Here's how the part is built. I have some questions about the finished solid (model axes, mm). A direction names the side the tool comes from. Coordinates: 2 decimals unless noted, no trailing zeros. Loops run counter-clockwise (first coordinate to the right, second up) from the corner with the lowest first, then second, coordinate; pieces in that order, holes last. Notation, with made-up numbers: (58, 7.25) -> (74, 7.25) arc R37 ccw to (74, 44.25) -> close; hole circle Ø10 at (7.25, 6). An arc over 180 degrees is marked (long way). Answer as a JSON object with one key per item and string values. Group by question number.
Q1. I want a section at A-A on x = 0. Write out the boundary of the cut face in (y, z) (3 decimals).
Q2. On a 3-axis mill with a long thin cutter (end or side, diameter ignored), from which of +Z, -Z, +X, -X, +Y, -Y can I reach the whole of each face in a straight line? I mean faces 4 (the flat face through (25.4, 70, 7)), 5 (the flat face through (0, 93, 7.5)), 6 (the flat face through (-1, -1, 13.625)). Say none if no direction works.
Q3. I need wall thicknesses on line 1 (Y direction, x = 11.25, z = 6.25); line 2 (Y direction, x = -1.5, z = 19.75); line 3 (Z direction, x = 12.5, y = -35) (3 decimals). Which ranges of each line are inside material? Lowest first, please.
Q4. I want a section at D-D on z = 5.75. Write out the boundary of the cut face in (x, y).
Q5. Thinking about a two-plate mould opening in Y: for faces 1 (the cylindrical face through (-1.71, -47.47, 18.56)), 2 (the cylindrical face through (-34.783, 18.75, 18.555)), 3 (the flat face through (-25.4, 70, 7)), which applies, released by +Y, released by -Y, zero draft, split by the parting line, or undercut?
Q6. I want a section at B-B on y = 18.64. Write out the boundary of the cut face in (x, z) (3 decimals).
Q7. I want a section at C-C on y = 37.28. Write out the boundary of the cut face in (x, z) (3 decimals), then the cut area to 3 significant figures.
Q8. I'm going to push flat-ended pins straight in: pin 1 (8 mm diameter, centred on x = 5.5, z = 10, fed in from -Y); pin 2 (11 mm diameter, centred on x = 1, z = 4, fed in from -Y); pin 3 (8 mm diameter, centred on x = -6.5, y = 8.5, fed in from -Z) (3 decimals); pin 4 (4.5 mm diameter, centred on x = -32.29, y = -18.64, fed in from -Z). Where does each tip first touch, or does it pass through?
```python
from build123d import *

# Parameters (mm, degrees)
SKETCH1_W           = 50.8
SKETCH1_H           = 65.000000038
SKETCH1_R           = 2.5
EXTRUDE_5_DEPTH     = 7.5
SKETCH1_3_W         = 50.8
SKETCH1_3_H         = 10
BOSS_EXTRUDE1_DEPTH = 13.625
BOSS_EXTRUDE2_START = 13.625
SKETCH1_4_R         = 2.5
SKETCH1_4_W         = 50.8
SKETCH1_4_H         = 10
BOSS_EXTRUDE2_DEPTH = 10
CHAMFER1_SIZE       = 10
CHAMFER1_SIZE_2     = 27.474774195
FILLET1_R           = 5


with BuildPart() as part:
    # Sketch1 → 5 (new body)
    with BuildSketch(Plane.XY):
        with Locations((0, 87.638385637)):
            Rectangle(SKETCH1_W, SKETCH1_H)
        with Locations((-11.25, 70.138385656)):
            Circle(SKETCH1_R, mode=Mode.SUBTRACT)
        with Locations((-11.25, 105.138385656)):
            Circle(SKETCH1_R, mode=Mode.SUBTRACT)
        with Locations((11.25, 70.138385656)):
            Circle(SKETCH1_R, mode=Mode.SUBTRACT)
        with Locations((11.25, 105.138385656)):
            Circle(SKETCH1_R, mode=Mode.SUBTRACT)
    extrude(amount=EXTRUDE_5_DEPTH)

    # Sketch1<3> → Boss-Extrude1 (add)
    with BuildSketch(Plane.XY):
        with Locations((0, 50.138385618)):
            Rectangle(SKETCH1_3_W, SKETCH1_3_H)
    extrude(amount=BOSS_EXTRUDE1_DEPTH)

    # Sketch1<4> → Boss-Extrude2 (add)
    # profile 1 of 2: a face of its own
    with BuildSketch(Plane.XY.offset(BOSS_EXTRUDE2_START)):
        with BuildLine():
            Line((-25.4, 45.138385618), (-25.4, 40.138385618))
            ThreePointArc((-25.4, 40.138385618), (0, -47.5), (25.4, 40.138385618))
            Line((25.4, 40.138385618), (25.4, 45.138385618))
            Line((25.4, 45.138385618), (-25.4, 45.138385618))
        make_face()
        with Locations((-32.285427053, -18.64)):
            Circle(SKETCH1_4_R, mode=Mode.SUBTRACT)
        with Locations((-32.285427053, 18.64)):
            Circle(SKETCH1_4_R, mode=Mode.SUBTRACT)
        with Locations((0, -37.28)):
            Circle(SKETCH1_4_R, mode=Mode.SUBTRACT)
        with Locations((32.285427053, -18.64)):
            Circle(SKETCH1_4_R, mode=Mode.SUBTRACT)
        with Locations((32.285427053, 18.64)):
            Circle(SKETCH1_4_R, mode=Mode.SUBTRACT)
        with Locations((0, 37.28)):
            Circle(SKETCH1_4_R, mode=Mode.SUBTRACT)
    # profile 2 of 2: a face of its own
    with BuildSketch(Plane.XY.offset(BOSS_EXTRUDE2_START)):
        with Locations((0, 50.138385618)):
            Rectangle(SKETCH1_4_W, SKETCH1_4_H)
    extrude(amount=BOSS_EXTRUDE2_DEPTH)

    # Chamfer1
    # the kernel refuses this chamfer: 27.474774195, 10 mm, written as the material it adds along each edge
    with BuildSketch(Plane(origin=(-25.4, 55.138385618, 7.5), x_dir=(0, 0.9950833631817486, -0.0990409022520505), z_dir=(1, 0, 0))) as chamfer1_piece_1_section:
        Polygon((CHAMFER1_SIZE * 0.995083363182, CHAMFER1_SIZE * 0.0990409022521), (-CHAMFER1_SIZE_2 * 0.0990409022504, CHAMFER1_SIZE_2 * 0.995083363165), (0, 0), align=None)
    chamfer1_piece_1 = extrude(amount=50.8, mode=Mode.PRIVATE)
    chamfer1_piece_1 = split(chamfer1_piece_1, bisect_by=Plane(origin=(0, 58.7545268, 23.625), z_dir=(0, 0, -1)), keep=Keep.TOP, mode=Mode.PRIVATE)
    add(chamfer1_piece_1)

    # Fillet1
    fillet1_edges = [part.edges().sort_by_distance(p)[0] for p in [
        (0, 59.26936559, 23.625),
    ]]
    fillet(fillet1_edges, radius=FILLET1_R)


solid = part.part
```
Result set:
{
 "1": {"outline": "(-47.5, 13.625) -> (-39.78, 13.625) -> (-39.78, 23.625) -> (-47.5, 23.625) -> close; (-34.78, 13.625) -> (34.78, 13.625) -> (34.78, 23.625) -> (-34.78, 23.625) -> close; (39.78, 13.625) -> (45.138, 13.625) -> (45.138, 0) -> (120.138, 0) -> (120.138, 7.5) -> (65.138, 7.5) -> (60.467, 20.335) arc R5 ccw to (55.768, 23.625) -> (39.78, 23.625) -> close"},
 "2": {"face 4": "+Z, -Z, +X, +Y", "face 5": "+Z, +X, -X, +Y", "face 6": "-Z, +X, -X, -Y"},
 "3": {"line 1": "y = 45.14 to 67.64, 72.64 to 102.64, 107.64 to 120.14", "line 2": "y = -47.48 to -39.28, -35.28 to 35.28, 39.28 to 60.68", "line 3": "z = 13.625 to 23.625"},
 "4": {"outline": "(-25.4, 45.14) -> (25.4, 45.14) -> (25.4, 120.14) -> (-25.4, 120.14) -> close; hole circle Ø5 at (-11.25, 70.14); hole circle Ø5 at (-11.25, 105.14); hole circle Ø5 at (11.25, 70.14); hole circle Ø5 at (11.25, 105.14)"},
 "5": {"face 1": "split by the parting line", "face 2": "undercut", "face 3": "zero draft"},
 "6": {"outline": "(-43.69, 13.625) -> (-34.785, 13.625) -> (-34.785, 23.625) -> (-43.69, 23.625) -> close; (-29.785, 13.625) -> (29.785, 13.625) -> (29.785, 23.625) -> (-29.785, 23.625) -> close; (34.785, 13.625) -> (43.69, 13.625) -> (43.69, 23.625) -> (34.785, 23.625) -> close"},
 "7": {"outline": "(-29.436, 13.625) -> (-2.5, 13.625) -> (-2.5, 23.625) -> (-29.436, 23.625) -> close; (2.5, 13.625) -> (29.436, 13.625) -> (29.436, 23.625) -> (2.5, 23.625) -> close", "area": "539 mm²"},
 "8": {"pin 1": "stops at y = -47.35", "pin 2": "stops at y = 45.14", "pin 3": "stops at z = 13.625", "pin 4": "passes through"}
}
